```python
from build123d import *

# Parameters (mm, degrees)
F1_DEPTH = 469.9
F3_DEPTH = 50.801


with BuildPart() as f1:
    # F0 (on Top) → F1 (new body)
    with BuildSketch(Plane.XY):
        with BuildLine():
            Line((22.225, 25.4), (-22.225, 25.4))
            ThreePointArc((-22.225, 25.4), (-24.470064, 24.470064), (-25.4, 22.225))
            Line((-25.4, 22.225), (-25.4, -22.225))
            ThreePointArc((-25.4, -22.225), (-24.470064, -24.470064), (-22.225, -25.4))
            Line((-22.225, -25.4), (22.225, -25.4))
            ThreePointArc((22.225, -25.4), (24.470064, -24.470064), (25.4, -22.225))
            Line((25.4, -22.225), (25.4, 22.225))
            ThreePointArc((25.4, 22.225), (24.470064, 24.470064), (22.225, 25.4))
        make_face()
        with BuildLine():
            ThreePointArc((-19.05, 17.4625), (-18.585032, 18.585032), (-17.4625, 19.05))
            Line((-17.4625, 19.05), (17.4625, 19.05))
            ThreePointArc((17.4625, 19.05), (18.585032, 18.585032), (19.05, 17.4625))
            Line((19.05, 17.4625), (19.05, -17.4625))
            ThreePointArc((19.05, -17.4625), (18.585032, -18.585032), (17.4625, -19.05))
            Line((17.4625, -19.05), (-17.4625, -19.05))
            ThreePointArc((-17.4625, -19.05), (-18.585032, -18.585032), (-19.05, -17.4625))
            Line((-19.05, -17.4625), (-19.05, 17.4625))
        make_face(mode=Mode.SUBTRACT)
    extrude(amount=F1_DEPTH)

    # F2 (on face) → F3 (cut, through all)
    with BuildSketch(Plane.YZ.offset(25.4)):
        Polygon((-25.4, 419.1), (25.4, 469.9), (-25.4, 469.9), align=None)
    extrude(amount=-F3_DEPTH, mode=Mode.SUBTRACT)


solid = f1.part
```
Design review of the part built by this model. Coordinates are the model's own, in mm. A direction names the side the tool comes from. Round coordinates to 2 decimals unless told otherwise and drop trailing zeros. Write each loop counter-clockwise with the first axis right and the second up, starting at its lowest first coordinate (ties: lowest second). Pieces come first, ordered by that corner, then holes. Notation, with made-up numbers: (13, -35) -> (20, -35) arc R9 ccw to (20, -23) -> close; hole circle Ø4 at (89, -23.5). An arc over 180 degrees is marked (long way). Answer in a Markdown table with one row per item.
Q1. For faces 1 (the face through (0, 19.05, 229)), 2 (the face through (0, -25.4, 207)), list the 3-axis set-ups (+Z, -Z, +X, -X, +Y, -Y) from which the entire face can be reached by the end or side of a thin tool; tool diameter is ignored.
The answers:
| item | result |
|---|---|
| face 1 | +Z, -Z |
| face 2 | +Z, -Z, +X, -X, -Y |
Q2. To check wall thickness, follow L1, parallel to X at y = -2, z = 131; L2, parallel to Z at x = 14, y = 19.5. State the ranges of each line that lie inside material, in increasing order. Write a range as [from, to].
The answers:
| item | result |
|---|---|
| L1 | [-25.4, -19.05], [19.05, 25.4] |
| L2 | [0, 464] |
Q3. Take a section at B-B, the plane x = 1. State the section outline as (y, z) points, then the cut area to 3 significant figures.
The answers:
| item | result |
|---|---|
| outline | (-25.4, 0) -> (-19.05, 0) -> (-19.05, 425.45) -> (-25.4, 419.1) -> close; (19.05, 0) -> (25.4, 0) -> (25.4, 469.9) -> (19.05, 463.55) -> close |
| area | 5,650 mm² |
Q4. Draft analysis for pull direction Y (two halves, no side actions). For faces 3 (the face through (0, 25.4, 232)), 4 (the face through (-19.05, 0, 228)), 5 (the face through (-22.2, -0.4, 444.1)), 6 (the face through (-25.4, 0, 230)), state which applies: +Y half, -Y half, draft (parallel to the pull), parting line (faces both ways), or undercut.
The answers:
| item | result |
|---|---|
| face 3 | +Y half |
| face 4 | undercut |
| face 5 | -Y half |
| face 6 | draft |
Q5. Take a section at A-A, the plane y = 10. State the section outline as (x, z) points, then the cut area to 3 significant figures.
The answers:
| item | result |
|---|---|
| outline | (-25.4, 0) -> (-19.05, 0) -> (-19.05, 454.5) -> (-25.4, 454.5) -> close; (19.05, 0) -> (25.4, 0) -> (25.4, 454.5) -> (19.05, 454.5) -> close |
| area | 5,770 mm² |
